Job drawing, mm, ordinate dimensions from the low corner. One solid piece. A direction names the side the tool comes from. Give positions to 0.01 mm unless a question says otherwise; leave off trailing zeros. Loops run counter-clockwise (first coordinate to the right, second up) from the corner with the lowest first, then second, coordinate; pieces in that order, holes last. Notation, with made-up numbers: M 69.25,-34 L 125.25,-34 A9 cw 125.25,-18 Z; hole C -10.5,66.5 d1. An arc over 180 degrees is marked long. Answer in a Markdown table with one row per item.
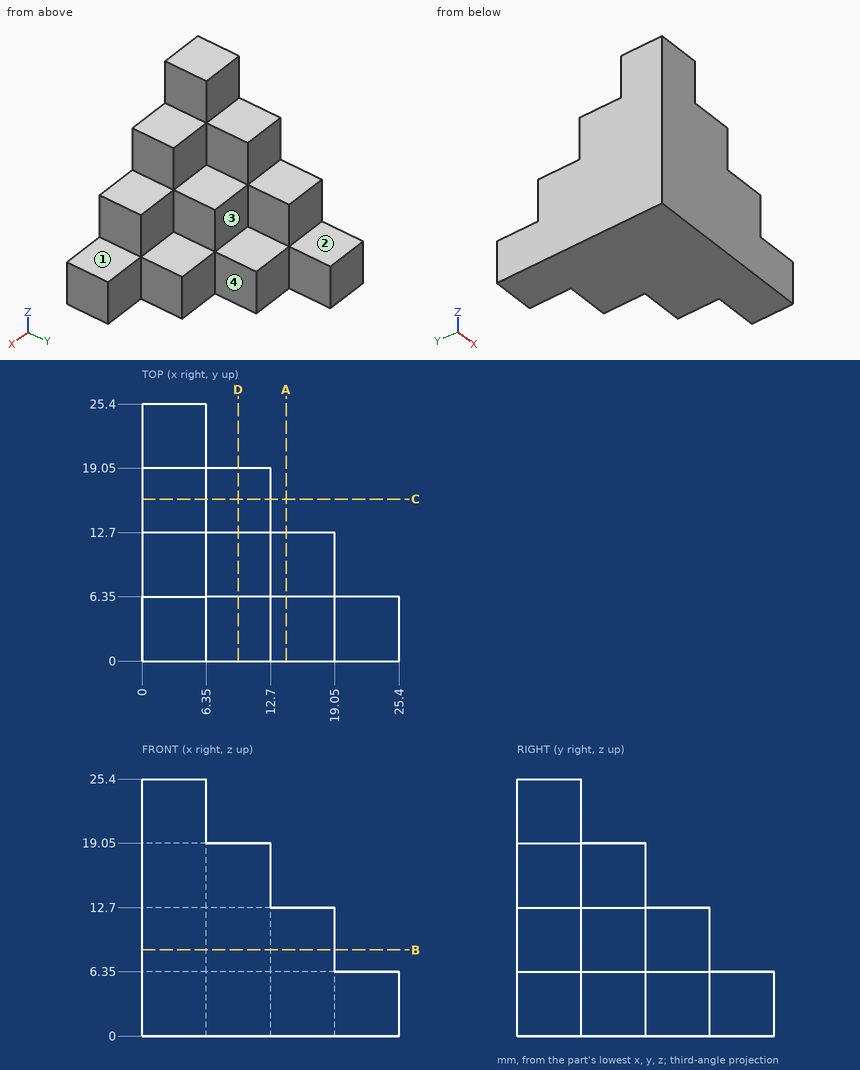
(1) Saw through at B-B (z = 8.5). Write the cut outline in (x, y).
Recorded:
| item | result |
|---|---|
| outline | M 0,0 L 19.05,0 L 19.05,6.35 L 12.7,6.35 L 12.7,12.7 L 6.35,12.7 L 6.35,19.05 L 0,19.05 Z |
(2) Which spindle directions (+Z, -Z, +X, -X, +Y, -Y) get a long thin tool onto all of the face, cutting with end or side? Do the marked faces 1, 2, 3 and 4. Say none if no direction does.
Recorded:
| item | result |
|---|---|
| face 1 | +Z, +X, +Y, -Y |
| face 2 | +Z, +X, -X, +Y |
| face 3 | +Z, +X, +Y |
| face 4 | +Z, -Z, +X, +Y |
(3) Pin check, flat tips, straight feed: pin 1 Ø5 at (y, z) = (22, 2.5) entering from +X; pin 2 Ø1 at (y, z) = (8.5, 5.5) entering from +X; pin 3 Ø5 at (x, y) = (22.5, 2) entering from +Z; pin 4 Ø5 at (x, z) = (14, 13.5) entering from -Y. Stop position of each tip, or through.
Recorded:
| item | result |
|---|---|
| pin 1 | stops at x = 6.35 |
| pin 2 | stops at x = 19.05 |
| pin 3 | stops at z = 6.35 |
| pin 4 | stops at y = 0 |
(4) Drill centre lines: line 1 along Z through (x, y) = (18.5, 9.25); line 2 along Z through (x, y) = (17, 6). Where is each one in solid material? Low to high.
Recorded:
| item | result |
|---|---|
| line 1 | z = 0 to 6.35 |
| line 2 | z = 0 to 12.7 |
(5) Saw through at A-A (x = 14.25). Write the cut outline in (y, z), plus the area to 3 significant figures.
Recorded:
| item | result |
|---|---|
| outline | M 0,0 L 12.7,0 L 12.7,6.35 L 6.35,6.35 L 6.35,12.7 L 0,12.7 Z |
| area | 121 mm^2 |
